from build123d import *

# Parameters (mm, degrees)
CYLINDER002_R          = 10
CYLINDER002_DEPTH      = 100
BOX001_W               = 2
BOX001_H               = 10
BOX001_DEPTH           = 10
PAD001_DEPTH           = 2
PAD_DEPTH              = 20
CUT001_PLACEMENT_ANGLE = 180


with BuildPart() as cylinder002:
    # Cylinder002 → Cylinder002 (new body)
    with BuildSketch(Plane(origin=(-48, 0, -17), x_dir=(0, 0, -1), z_dir=(1, 0, 0))):
        Circle(CYLINDER002_R)
    extrude(amount=CYLINDER002_DEPTH)


with BuildPart() as cube001:
    # Box001 → Box001 (new body)
    with BuildSketch(Plane(origin=(-1, -63, -13), x_dir=(1, 0, 0), z_dir=(0, 0, 1))):
        with Locations((1, 5)):
            Rectangle(BOX001_W, BOX001_H)
    extrude(amount=BOX001_DEPTH)


with BuildPart() as body001:
    # Sketch001 → Pad001 (new body)
    with BuildSketch(Plane.XY):
        with BuildLine():
            ThreePointArc((32.166162, 22.5), (0, 54.666162), (-32.166162, 22.5))
            Line((-32.166162, 22.5), (-32.166162, -22.5))
            ThreePointArc((-32.166162, -22.5), (0, -54.666162), (32.166162, -22.5))
            Line((32.166162, 22.5), (32.166162, -22.5))
        make_face()
        Polygon((-17, 27), (0, 46.672316), (17, 27), (7, 27), (7, 6), (-7, 6), (-7, 27), align=None, mode=Mode.SUBTRACT)
        Polygon((-20.337316, -16), (-20.337316, -30), (0.662684, -30), (0.662684, -40), (20.335, -23), (0.662684, -6), (0.662684, -16), align=None, mode=Mode.SUBTRACT)
    extrude(amount=PAD001_DEPTH)


with BuildPart() as f_64_trafficlightcasetop:
    # Sketch → Pad (new body)
    with BuildSketch(Plane.XY):
        with BuildLine():
            ThreePointArc((34.15435, 22.5), (0, 56.65435), (-34.15435, 22.5))
            Line((-34.15435, 22.5), (-34.15435, -22.5))
            ThreePointArc((-34.15435, -22.5), (0, -56.65435), (34.15435, -22.5))
            Line((34.15435, 22.5), (34.15435, -22.5))
        make_face()
        with BuildLine():
            ThreePointArc((32.15435, 22.5), (0, 54.65435), (-32.15435, 22.5))
            Line((-32.15435, 22.5), (-32.15435, -22.5))
            ThreePointArc((-32.15435, -22.5), (0, -54.65435), (32.15435, -22.5))
            Line((32.15435, 22.5), (32.15435, -22.5))
        make_face(mode=Mode.SUBTRACT)
    extrude(amount=PAD_DEPTH)


with BuildPart() as f_64_trafficlightcasetop_1:
    # Body placement: moved
    add(f_64_trafficlightcasetop.part.moved(Location((0, 0, -18))))

    # Fusion: union Body001
    add(body001.part)

    # Cut001: cut Cube001
    add(cube001.part, mode=Mode.SUBTRACT)


with BuildPart() as f_64_trafficlightcasetop_2:
    # Cut001 placement: moved
    add(f_64_trafficlightcasetop_1.part.rotate(Axis((0, 0, 0), (0, 0, 1)), CUT001_PLACEMENT_ANGLE))

    # Cut004: cut Cylinder002
    add(cylinder002.part, mode=Mode.SUBTRACT)


solid = f_64_trafficlightcasetop_2.part
Source: CAD feature listing. Evaluate the final solid. Frame: model axes, mm. A direction names the side the tool comes from. Give positions to 0.01 mm unless a question says otherwise; leave off trailing zeros. Write each loop counter-clockwise with the first axis right and the second up, starting at its lowest first coordinate (ties: lowest second). Pieces come first, ordered by that corner, then holes. Notation, with made-up numbers: (-7, -10.5) -> (41, -10.5) arc R20 cw to (41, -1.5) -> close; hole circle Ø4 at (24, 14.5). An arc over 180 degrees is marked (long way). Return JSON: item names as keys, results as strings. Group by question number.
1. Section C-C, the plane y = 0. Output: boundary loops of the cut face in (x, z).
2. Section B-B, the plane z = -8.75. Output: boundary loops of the cut face in (x, y), then the cut area to 3 significant figures.
3. Mould query, pull axis X, two halves, no side actions, for faces 4 (the face through (33, 0, -7)), 5 (the face through (-34.154, 0, -6)), 6 (the face through (32.154, 0, -5)). Classes: +X half, -X half, draft (parallel to the pull), parting line (faces both ways), or undercut.
4. Pin query (flat end, axial travel): pin 1 Ø1.6 at (x, z) = (-10.5, 0.5) entering from -Y; pin 2 Ø12 at (y, z) = (0, -17) entering from +X; pin 3 Ø8 at (x, y) = (-12.5, 36.5) entering from -Z; pin 4 Ø0.6 at (y, z) = (35, 1) entering from -X. Return the tip coordinate at first contact, or that it passes through.
5. Section A-A, the plane y = -13. Output: boundary loops of the cut face in (x, z).
6. Material intervals for line 1 (X direction, y = 9, z = -6.25); line 2 (Y direction, x = -23, z = -9.5); line 3 (Y direction, x = -22, z = -6.5), sorted ascending. Write a range as from..to.
7. Access query for faces 1 (the face through (0, -1, 0)), 2 (the face through (0.751, 56.646, -14.807)), 3 (the face through (8.62, -36.7, 0.99)). Directions: +Z, -Z, +X, -X, +Y, -Y. A direction counts if a zero-diameter tool reaches every point of the face in a straight line with its end or side. Return the directions, or none.
8. Section D-D, the plane x = -11. Output: boundary loops of the cut face in (y, z).
Determined:
{
 "1": {"outline": "(-34.15, -7) -> (-32.15, -7) -> (-32.15, 0) -> (32.15, 0) -> (32.15, -7) -> (34.15, -7) -> (34.15, 2) -> (-34.15, 2) -> close"},
 "2": {"outline": "(-34.15, -22.5) arc R34.15 ccw to (34.15, -22.5) -> (34.15, -5.65) -> (32.15, -5.65) -> (32.15, -22.5) arc R32.15 cw to (-32.15, -22.5) -> (-32.15, -5.65) -> (-34.15, -5.65) -> close; (-34.15, 5.65) -> (-32.15, 5.65) -> (-32.15, 22.5) arc R32.15 cw to (-1, 54.64) -> (-1, 56.64) arc R34.15 ccw to (-34.15, 22.5) -> close; (1, 54.64) arc R32.15 cw to (32.15, 22.5) -> (32.15, 5.65) -> (34.15, 5.65) -> (34.15, 22.5) arc R34.15 ccw to (1, 56.64) -> close", "area": "547 mm2"},
 "3": {"face 4": "draft", "face 5": "-X half", "face 6": "undercut"},
 "4": {"pin 1": "stops at y = -55.25", "pin 2": "passes through", "pin 3": "stops at z = 0", "pin 4": "stops at x = -31.9"},
 "5": {"outline": "(-34.15, -18) -> (-32.15, -18) -> (-32.15, 0) -> (-7, 0) -> (-7, 2) -> (-34.15, 2) -> close; (7, 0) -> (32.15, 0) -> (32.15, -18) -> (34.15, -18) -> (34.15, 2) -> (7, 2) -> close"},
 "6": {"line 1": "x = -34.15..-32.15, 32.15..34.15", "line 2": "y = -47.75..-44.97, 44.97..47.75", "line 3": "y = -48.63..-45.95, 45.95..48.63"},
 "7": {"face 1": "-Z", "face 2": "+Z, -Z, +Y", "face 3": "+Z, -Z"},
 "8": {"outline": "(-54.83, -18) -> (-52.71, -18) -> (-52.71, 0) -> (-33.94, 0) -> (-33.94, 2) -> (-54.83, 2) -> close; (-27, 0) -> (14.93, 0) -> (14.93, 2) -> (-27, 2) -> close; (31.07, 0) -> (52.71, 0) -> (52.71, -18) -> (54.83, -18) -> (54.83, 2) -> (31.07, 2) -> close"}
}
